Build history of the part. All positions in model axes, mm. A direction names the side the tool comes from. Round coordinates to 2 decimals unless told otherwise and drop trailing zeros. Write each loop counter-clockwise with the first axis right and the second up, starting at its lowest first coordinate (ties: lowest second). Pieces come first, ordered by that corner, then holes. Notation, with made-up numbers: (22, -25.75) -> (68, -25.75) arc R34 ccw to (68, 8.25) -> close; hole circle Ø5 at (41, 84). An arc over 180 degrees is marked (long way). Answer in a Markdown table with one row per item.
```python
from build123d import *

# Parameters (mm, degrees)
BOSS_EXTRUDE1_DEPTH                          = 4
CUT_EXTRUDE1_REACH                           = 222.744
SKETCH2_W                                    = 4
SKETCH2_H                                    = 50
CSK_FOR_M4_COUNTERSUNK_FLAT_HEAD_SCR_2_COUNT = 2
CSK_FOR_M4_COUNTERSUNK_FLAT_HEAD_SCR_2_PITCH = 148
CSK_FOR_M4_COUNTERSUNK_FLAT_HEAD_SCR_3_COUNT = 2
CSK_FOR_M4_COUNTERSUNK_FLAT_HEAD_SCR_3_PITCH = 168.237926759
CSK_FOR_M4_COUNTERSUNK_FLAT_HEAD_SCR_4_COUNT = 2
CSK_FOR_M4_COUNTERSUNK_FLAT_HEAD_SCR_4_PITCH = 80
CUT_EXTRUDE2_REACH                           = 222.744


with BuildPart() as part:
    # Sketch1 → Boss-Extrude1 (new body)
    with BuildSketch(Plane.XY):
        Polygon((0, 25), (0, 0), (214, 0), (214, 54), (119, 54), (119, 50), (69, 50), (69, 54), (4, 54), (4, 25), align=None)
        Polygon((0, 0), (0, -25), (4, -25), (4, -54), (69, -54), (69, -50), (119, -50), (119, -54), (214, -54), (214, 0), align=None)
    extrude(amount=BOSS_EXTRUDE1_DEPTH)

    # Sketch2 → Cut-Extrude1 (cut, up to next)
    with BuildSketch(Plane.XY.offset(4), mode=Mode.PRIVATE) as cut_extrude1_sk1:
        with Locations((174, 0)):
            Rectangle(SKETCH2_W, SKETCH2_H)
    cut_extrude1_tool1 = extrude(cut_extrude1_sk1.sketch, amount=-CUT_EXTRUDE1_REACH, mode=Mode.PRIVATE) & part.part
    add(cut_extrude1_tool1.solids().sort_by_distance((174, 0, 4))[0], mode=Mode.SUBTRACT)

    # Sketch4 → CSK for M4 Countersunk Flat Head Screw1 (revolve, cut)
    with BuildSketch(Plane(origin=(14, 40, 4), x_dir=(0, -1, 0), z_dir=(1, 0, 0))):
        Polygon((0, 0), (0, 4), (2.25, 4), (2.25, 2.45), (4.7, 0), align=None)
    csk_for_m4_countersunk_flat_head_screw1 = revolve(axis=Axis((14, 40, 10.35), (0, 0, -1)), mode=Mode.SUBTRACT)

    # CSK for M4 Countersunk Flat Head Scr 2: CSK for M4 Countersunk Flat Head Screw1 ×2
    with Locations(*[(i * CSK_FOR_M4_COUNTERSUNK_FLAT_HEAD_SCR_2_PITCH, 0, 0) for i in range(1, CSK_FOR_M4_COUNTERSUNK_FLAT_HEAD_SCR_2_COUNT)]):
        add(csk_for_m4_countersunk_flat_head_screw1, mode=Mode.SUBTRACT)

    # CSK for M4 Countersunk Flat Head Scr 3: CSK for M4 Countersunk Flat Head Screw1 ×2
    with Locations(*[Vector(0.8797065135761271, -0.47551703436547405, 0) * (i * CSK_FOR_M4_COUNTERSUNK_FLAT_HEAD_SCR_3_PITCH) for i in range(1, CSK_FOR_M4_COUNTERSUNK_FLAT_HEAD_SCR_3_COUNT)]):
        add(csk_for_m4_countersunk_flat_head_screw1, mode=Mode.SUBTRACT)

    # CSK for M4 Countersunk Flat Head Scr 4: CSK for M4 Countersunk Flat Head Screw1 ×2
    with Locations(*[(0, -i * CSK_FOR_M4_COUNTERSUNK_FLAT_HEAD_SCR_4_PITCH, 0) for i in range(1, CSK_FOR_M4_COUNTERSUNK_FLAT_HEAD_SCR_4_COUNT)]):
        add(csk_for_m4_countersunk_flat_head_screw1, mode=Mode.SUBTRACT)

    # Sketch5 → Cut-Extrude2 (cut, up to next)
    with BuildSketch(Plane(origin=(0, 0, 0), x_dir=(-1, 0, 0), z_dir=(0, 0, -1)), mode=Mode.PRIVATE) as cut_extrude2_sk1:
        with BuildLine():
            Line((-122.777043469, 25), (-122.777043469, -25))
            ThreePointArc((-122.777043469, -25), (-125.777043469, -28), (-128.777043469, -25))
            Line((-128.777043469, -25), (-128.777043469, 25))
            ThreePointArc((-128.777043469, 25), (-125.777043469, 28), (-122.777043469, 25))
        make_face()
    cut_extrude2_tool1 = extrude(cut_extrude2_sk1.sketch, amount=-CUT_EXTRUDE2_REACH, mode=Mode.PRIVATE) & part.part
    # Sketch5 → Cut-Extrude2 (cut, up to next)
    with BuildSketch(Plane(origin=(0, 0, 0), x_dir=(-1, 0, 0), z_dir=(0, 0, -1)), mode=Mode.PRIVATE) as cut_extrude2_sk2:
        with BuildLine():
            Line((-113.777043469, 25), (-113.777043469, -25))
            ThreePointArc((-113.777043469, -25), (-110.777043469, -28), (-107.777043469, -25))
            Line((-107.777043469, -25), (-107.777043469, 25))
            ThreePointArc((-107.777043469, 25), (-110.777043469, 28), (-113.777043469, 25))
        make_face()
    cut_extrude2_tool2 = extrude(cut_extrude2_sk2.sketch, amount=-CUT_EXTRUDE2_REACH, mode=Mode.PRIVATE) & part.part
    # Sketch5 → Cut-Extrude2 (cut, up to next)
    with BuildSketch(Plane(origin=(0, 0, 0), x_dir=(-1, 0, 0), z_dir=(0, 0, -1)), mode=Mode.PRIVATE) as cut_extrude2_sk3:
        with BuildLine():
            Line((-98.777043469, 25), (-98.777043469, -25))
            ThreePointArc((-98.777043469, -25), (-95.777043469, -28), (-92.777043469, -25))
            Line((-92.777043469, -25), (-92.777043469, 25))
            ThreePointArc((-92.777043469, 25), (-95.777043469, 28), (-98.777043469, 25))
        make_face()
    cut_extrude2_tool3 = extrude(cut_extrude2_sk3.sketch, amount=-CUT_EXTRUDE2_REACH, mode=Mode.PRIVATE) & part.part
    # Sketch5 → Cut-Extrude2 (cut, up to next)
    with BuildSketch(Plane(origin=(0, 0, 0), x_dir=(-1, 0, 0), z_dir=(0, 0, -1)), mode=Mode.PRIVATE) as cut_extrude2_sk4:
        with BuildLine():
            Line((-83.777043469, 25), (-83.777043469, -25))
            ThreePointArc((-83.777043469, -25), (-80.777043469, -28), (-77.777043469, -25))
            Line((-77.777043469, -25), (-77.777043469, 25))
            ThreePointArc((-77.777043469, 25), (-80.777043469, 28), (-83.777043469, 25))
        make_face()
    cut_extrude2_tool4 = extrude(cut_extrude2_sk4.sketch, amount=-CUT_EXTRUDE2_REACH, mode=Mode.PRIVATE) & part.part
    add(cut_extrude2_tool1.solids().sort_by_distance((125.777043, 0, 0))[0], mode=Mode.SUBTRACT)
    add(cut_extrude2_tool2.solids().sort_by_distance((110.777043, 0, 0))[0], mode=Mode.SUBTRACT)
    add(cut_extrude2_tool3.solids().sort_by_distance((95.777043, 0, 0))[0], mode=Mode.SUBTRACT)
    add(cut_extrude2_tool4.solids().sort_by_distance((80.777043, 0, 0))[0], mode=Mode.SUBTRACT)


solid = part.part
```
Q1. Two-plate mould, pull along X, no slides. Class faces 1 (the flat face through (4, 40, 2)), 2 (the flat face through (92.777, 0, 2)), 3 (the flat face through (176, 0, 2)), 4 (the flat face through (214, -1, 2)): released by +X, released by -X, zero draft, split by the parting line, or undercut.
A:
| item | result |
|---|---|
| face 1 | released by -X |
| face 2 | undercut |
| face 3 | undercut |
| face 4 | released by +X |
Q2. Saw through at B-B on y = -40. Write the cut outline in (x, z), plus the area to 3 significant figures.
A:
| item | result |
|---|---|
| outline | (4, 0) -> (11.75, 0) -> (11.75, 1.55) -> (9.3, 4) -> (4, 4) -> close; (16.25, 0) -> (159.75, 0) -> (159.75, 1.55) -> (157.3, 4) -> (18.7, 4) -> (16.25, 1.55) -> close; (164.25, 0) -> (214, 0) -> (214, 4) -> (166.7, 4) -> (164.25, 1.55) -> close |
| area | 792 mm² |
Q3. Wall check: line 1 (X direction, y = 40, z = 0.65); line 2 (X direction, y = -20.5, z = 3.2); line 3 (Y direction, x = 14, z = 0.95). Give the ranges that are in metal, low to high. Write a range as [from, to].
A:
| item | result |
|---|---|
| line 1 | [4, 11.75], [16.25, 159.75], [164.25, 214] |
| line 2 | [0, 77.78], [83.78, 92.78], [98.78, 107.78], [113.78, 122.78], [128.78, 172], [176, 214] |
| line 3 | [-54, -42.25], [-37.75, 37.75], [42.25, 54] |
Q4. Saw through at D-D on z = 0.65. State how many separate pieces and enclosed holes the cut face has, plus the area to 3 significant figures.
A:
| item | result |
|---|---|
| separate pieces | 1 |
| enclosed holes | 9 |
| area | 20,900 mm² |
Q5. Saw through at A-A on x = 162. Write the cut outline in (y, z), plus the area to 3 significant figures.
A:
| item | result |
|---|---|
| outline | (-54, 0) -> (-42.25, 0) -> (-42.25, 1.55) -> (-44.7, 4) -> (-54, 4) -> close; (-37.75, 0) -> (37.75, 0) -> (37.75, 1.55) -> (35.3, 4) -> (-35.3, 4) -> (-37.75, 1.55) -> close; (42.25, 0) -> (54, 0) -> (54, 4) -> (44.7, 4) -> (42.25, 1.55) -> close |
| area | 384 mm² |
Q6. Saw through at C-C on y = 19. Write the cut outline in (x, z).
A:
| item | result |
|---|---|
| outline | (0, 0) -> (77.78, 0) -> (77.78, 4) -> (0, 4) -> close; (83.78, 0) -> (92.78, 0) -> (92.78, 4) -> (83.78, 4) -> close; (98.78, 0) -> (107.78, 0) -> (107.78, 4) -> (98.78, 4) -> close; (113.78, 0) -> (122.78, 0) -> (122.78, 4) -> (113.78, 4) -> close; (128.78, 0) -> (172, 0) -> (172, 4) -> (128.78, 4) -> close; (176, 0) -> (214, 0) -> (214, 4) -> (176, 4) -> close |
Q7. Which spindle directions (+Z, -Z, +X, -X, +Y, -Y) get a long thin tool onto all of the face, cutting with end or side? Do faces 5 (the flat face through (174, -25, 2)), 6 (the flat face through (2, -25, 2)), 7 (the flat face through (119, -52, 2)). Say none if no direction does.
A:
| item | result |
|---|---|
| face 5 | +Z, -Z |
| face 6 | +Z, -Z, -X, -Y |
| face 7 | +Z, -Z, -Y |
Q8. Drop flat-ended pins along their axis: P1, Ø5, axis at x = 14, y = -40, coming from the +Z side; P2, Ø1.2, axis at x = 1, z = 1.5, coming from the -Y side; P3, Ø1.2, axis at y = 51.5, z = 1.5, coming from the -X side. Give the stop position or say it passes through.
A:
| item | result |
|---|---|
| P1 | z = 1.8 |
| P2 | y = -25 |
| P3 | x = 4 |
